from build123d import *

# Parameters (mm, degrees)
F3_R     = 2.75
F4_DEPTH = 3
F6_DEPTH = 1.5
F7_R     = 1.5
F8_DEPTH = 12
F9_SIZE  = 0.15
F10_SIZE = 0.3


with BuildPart() as f4:
    # F3 (on Top) → F4 (new body)
    with BuildSketch(Plane.XY):
        Circle(F3_R)
    extrude(amount=F4_DEPTH)

    # F5 (on face) → F6 (cut)
    with BuildSketch(Plane(origin=(0, 0, 0), x_dir=(1, 0, 0), z_dir=(0, 0, -1))):
        Polygon((0.7216878365, 1.25), (-0.7216878365, 1.25), (-1.443375673, 0), (-0.7216878365, -1.25), (0.7216878365, -1.25), (1.443375673, 0), align=None)
    extrude(amount=-F6_DEPTH, mode=Mode.SUBTRACT)

    # F7 (on face) → F8 (join)
    with BuildSketch(Plane.XY.offset(3)):
        Circle(F7_R)
    extrude(amount=F8_DEPTH)

    # F9
    f9_edges = [f4.edges().sort_by_distance(p)[0] for p in [
        (-2.75, 0, 0),
        (0, -1.25, 0),
        (1.082532, -0.625, 0),
        (1.082532, 0.625, 0),
        (0, 1.25, 0),
        (-1.082532, -0.625, 0),
        (-1.082532, 0.625, 0),
    ]]
    chamfer(f9_edges, length=F9_SIZE)

    # F10
    f10_edges = [f4.edges().sort_by_distance(p)[0] for p in [
        (-1.5, 0, 15),
    ]]
    chamfer(f10_edges, length=F10_SIZE)


solid = f4.part
Verification items for the finished model (mm, model axes). A direction names the side the tool comes from. Coordinates: 2 decimals unless noted, no trailing zeros. Loops run counter-clockwise (first coordinate to the right, second up) from the corner with the lowest first, then second, coordinate; pieces in that order, holes last. Notation, with made-up numbers: (85, 10.25) -> (96, 10.25) arc R34 cw to (96, 41.25) -> close; hole circle Ø4 at (72, -22.75). An arc over 180 degrees is marked (long way). Write each question's results on one line, items separated by ' | '.
Item 1: Tool access check on faces 5 (the face through (0, 0, 1.5)), 6 (the face through (1.2, -1.2, 3)), 7 (the face through (0, 0, 15)). Record the directions out of +Z, -Z, +X, -X, +Y, -Y that give a thin tool (end or side, any length) a straight path to the whole face; none if there is none.
Found:
face 5: -Z | face 6: +Z | face 7: +Z, +X, -X, +Y, -Y
Item 2: Section check A-A, the plane x = 0. Enter the section's corners in (y, z), plus the area to 3 significant figures.
Found:
outline: (-2.75, 0.15) -> (-2.6, 0) -> (-1.4, 0) -> (-1.25, 0.15) -> (-1.25, 1.5) -> (1.25, 1.5) -> (1.25, 0.15) -> (1.4, 0) -> (2.6, 0) -> (2.75, 0.15) -> (2.75, 3) -> (1.5, 3) -> (1.5, 14.7) -> (1.2, 15) -> (-1.2, 15) -> (-1.5, 14.7) -> (-1.5, 3) -> (-2.75, 3) -> close | area: 48.6 mm2
Item 3: Gauge pin test, flat ends, axial feed: pin 1 (1.2 mm diameter, centred on x = 0.5, y = 0.5, fed in from -Z); pin 2 (1.5 mm diameter, centred on x = -1, z = 2.5, fed in from +Y); pin 3 (1 mm diameter, centred on y = 1, z = 9.5, fed in from -X). Record the tip position at first contact, or that the pin passes through.
Found:
pin 1: stops at z = 0.12 | pin 2: stops at y = 2.74 | pin 3: stops at x = -1.41
Item 4: Section check B-B, the plane z = 8.5. Enter the section's corners in (x, y).
Found:
outline: circle Ø3 at (0, 0)
Item 5: Mould release check, pull along Y, two halves, no side actions. Record for faces 1 (the face through (-1.5, 0.07, 8.77)), 2 (the face through (2, 0, 0)), 3 (the face through (1.088, -0.616, 0.816)), 4 (the face through (1.08, 0.63, 0.82)): +Y half, -Y half, draft (parallel to the pull), parting line (faces both ways), or undercut.
Found:
face 1: parting line | face 2: draft | face 3: undercut | face 4: undercut
Item 6: Material ranges on L1, parallel to Z at x = -0.9, y = 1.9; L2, parallel to Y at x = -0.4, z = 9; L3, parallel to Z at x = -1.1, y = -0.25, recorded low to high.
Found:
L1: z = 0 to 3 | L2: y = -1.45 to 1.45 | L3: z = 1.5 to 15
